For this review, take the finished solid that the model builds, in its own axes (mm). A direction names the side the tool comes from. Coordinates: 2 decimals unless noted, no trailing zeros. Loops run counter-clockwise (first coordinate to the right, second up) from the corner with the lowest first, then second, coordinate; pieces in that order, holes last. Notation, with made-up numbers: (26, 23.25) -> (74, 23.25) arc R23 ccw to (74, 59.25) -> close; hole circle Ø11 at (9.5, -30). An arc over 180 degrees is marked (long way). Answer in a Markdown table with one row per item.
from build123d import *
from build123d import SkipClean  # not in build123d's __all__

# Parameters (mm, degrees)
F1_DEPTH  = 10
F2_DEPTH  = 12.5
F3_DEPTH  = 10.3
F4_R      = 1.5
F5_DEPTH  = 2
F4_R_2    = 1.55
F6_DEPTH  = 5
F7_R      = 1.5
F8_DEPTH  = 2
F7_R_2    = 1.55
F9_DEPTH  = 5
F11_DEPTH = 12.5


with BuildPart() as f1:
    # F0 (on Front) → F1 (new body, symmetric)
    with BuildSketch(Plane.XZ):
        with BuildLine():
            ThreePointArc((0, -3.75), (2.6516504294, -2.6516504294), (3.75, 0))
            ThreePointArc((3.75, 0), (2.6516504294, 2.6516504294), (0, 3.75))
            ThreePointArc((0, 3.75), (-2.6516504294, 2.6516504294), (-3.75, 0))
            ThreePointArc((-3.75, 0), (-2.6516504294, -2.6516504294), (0, -3.75))
        make_face()
        with BuildLine():
            ThreePointArc((0, 3.75), (2.6516504294, 2.6516504294), (3.75, 0))
            ThreePointArc((3.75, 0), (4.8483495706, 2.6516504294), (7.5, 3.75))
            Line((7.5, 3.75), (0, 3.75))
        make_face()
        with BuildLine():
            ThreePointArc((7.5, 3.75), (4.8483495706, 2.6516504294), (3.75, 0))
            ThreePointArc((3.75, 0), (4.8483495706, -2.6516504294), (7.5, -3.75))
            ThreePointArc((7.5, -3.75), (10.1516504294, -2.6516504294), (11.25, 0))
            ThreePointArc((11.25, 0), (10.1516504294, 2.6516504294), (7.5, 3.75))
        make_face()
        with BuildLine():
            ThreePointArc((7.5, -3.75), (4.8483495706, -2.6516504294), (3.75, 0))
            ThreePointArc((3.75, 0), (2.6516504294, -2.6516504294), (0, -3.75))
            Line((0, -3.75), (7.5, -3.75))
        make_face()
    extrude(amount=F1_DEPTH, both=True)

    # F0 (on Front) → F2 (join, symmetric)
    with BuildSketch(Plane.XZ):
        with BuildLine():
            ThreePointArc((-7.5, -3.75), (-4.8483495706, -2.6516504294), (-3.75, 0))
            ThreePointArc((-3.75, 0), (-4.8483495706, 2.6516504294), (-7.5, 3.75))
            ThreePointArc((-7.5, 3.75), (-11.25, 0), (-7.5, -3.75))
        make_face()
        with BuildLine():
            ThreePointArc((-3.75, 0), (-2.6516504294, 2.6516504294), (0, 3.75))
            Line((0, 3.75), (-7.5, 3.75))
            ThreePointArc((-7.5, 3.75), (-4.8483495706, 2.6516504294), (-3.75, 0))
        make_face()
        with BuildLine():
            ThreePointArc((0, -3.75), (2.6516504294, -2.6516504294), (3.75, 0))
            ThreePointArc((3.75, 0), (2.6516504294, 2.6516504294), (0, 3.75))
            ThreePointArc((0, 3.75), (-2.6516504294, 2.6516504294), (-3.75, 0))
            ThreePointArc((-3.75, 0), (-2.6516504294, -2.6516504294), (0, -3.75))
        make_face()
        with BuildLine():
            Line((-7.5, -3.75), (0, -3.75))
            ThreePointArc((0, -3.75), (-2.6516504294, -2.6516504294), (-3.75, 0))
            ThreePointArc((-3.75, 0), (-4.8483495706, -2.6516504294), (-7.5, -3.75))
        make_face()
    extrude(amount=F2_DEPTH, both=True)

    # F0 (on Front) → F3 (cut, symmetric)
    with BuildSketch(Plane.XZ):
        with BuildLine():
            ThreePointArc((-7.5, -3.75), (-4.8483495706, -2.6516504294), (-3.75, 0))
            ThreePointArc((-3.75, 0), (-4.8483495706, 2.6516504294), (-7.5, 3.75))
            ThreePointArc((-7.5, 3.75), (-11.25, 0), (-7.5, -3.75))
        make_face()
        with BuildLine():
            Line((-7.5, -3.75), (0, -3.75))
            ThreePointArc((0, -3.75), (-2.6516504294, -2.6516504294), (-3.75, 0))
            ThreePointArc((-3.75, 0), (-4.8483495706, -2.6516504294), (-7.5, -3.75))
        make_face()
        with BuildLine():
            ThreePointArc((-3.75, 0), (-2.6516504294, 2.6516504294), (0, 3.75))
            Line((0, 3.75), (-7.5, 3.75))
            ThreePointArc((-7.5, 3.75), (-4.8483495706, 2.6516504294), (-3.75, 0))
        make_face()
    with SkipClean():  # cleaning this boolean's faces spoils the solid; the shape is the same uncleaned
        extrude(amount=F3_DEPTH, both=True, mode=Mode.SUBTRACT)

    # F4 (on face) → F5 (join)
    with BuildSketch(Plane.XZ.offset(10)):
        with Locations((7.5, 0)):
            Circle(F4_R)
    extrude(amount=F5_DEPTH)

    # F4 (on face) → F6 (cut)
    with BuildSketch(Plane.XZ.offset(10)):
        with Locations((-7.4913557619, 0)):
            Circle(F4_R_2)
    extrude(amount=F6_DEPTH, mode=Mode.SUBTRACT)

    # F7 (on face) → F8 (join)
    with BuildSketch(Plane(origin=(0, 10, 0), x_dir=(-1, 0, 0), z_dir=(0, 1, 0))):
        with Locations((-7.5, 0)):
            Circle(F7_R)
    extrude(amount=F8_DEPTH)

    # F7 (on face) → F9 (cut)
    with BuildSketch(Plane(origin=(0, 10, 0), x_dir=(-1, 0, 0), z_dir=(0, 1, 0))):
        with Locations((7.4891448021, 0)):
            Circle(F7_R_2)
    extrude(amount=F9_DEPTH, mode=Mode.SUBTRACT)

    # F10 (on Top) → F11 (cut, symmetric)
    with BuildSketch(Plane.XY):
        Polygon((-3.2, -10.3), (-3.2, 0), (-3.2, 10.3), (-14.7820527132, 10.3), (-14.7820527132, -10.3), align=None)
    extrude(amount=F11_DEPTH, both=True, mode=Mode.SUBTRACT)


solid = f1.part
Item 1: The part is to be moulded in two halves that separate along Y. For faces 5 (the flat face through (-3.2, 0, 0)), 6 (the flat face through (5.5, 10, 0.1)), 7 (the flat face through (-4, 11, -3.75)), say which applies: +Y half, -Y half, draft (parallel to the pull), parting line (faces both ways), or undercut.
Worked answers:
| item | result |
|---|---|
| face 5 | undercut |
| face 6 | +Y half |
| face 7 | draft |
Item 2: For faces 1 (the flat face through (-4, -11, -3.75)), 2 (the cylindrical face through (9, 11, 0)), 3 (the cylindrical face through (6, -11, 0)), 4 (the flat face through (7, -12, 0)), list the 3-axis set-ups (+Z, -Z, +X, -X, +Y, -Y) from which the entire face can be reached by the end or side of a thin tool; tool diameter is ignored.
Worked answers:
| item | result |
|---|---|
| face 1 | -Z, +X, -X, +Y, -Y |
| face 2 | +Y |
| face 3 | -Y |
| face 4 | +Z, -Z, +X, -Y |
Item 3: Take a section at A-A, the plane z = 0.75. State the section outline as (x, y) points.
Worked answers:
| item | result |
|---|---|
| outline | (-11.17, -12.5) -> (-8.85, -12.5) -> (-8.85, -10.3) -> (-11.17, -10.3) -> close; (-11.17, 10.3) -> (-8.85, 10.3) -> (-8.85, 12.5) -> (-11.17, 12.5) -> close; (-6.13, -12.5) -> (3.67, -12.5) -> (3.67, -10) -> (6.2, -10) -> (6.2, -12) -> (8.8, -12) -> (8.8, -10) -> (11.17, -10) -> (11.17, 10) -> (8.8, 10) -> (8.8, 12) -> (6.2, 12) -> (6.2, 10) -> (3.67, 10) -> (3.67, 12.5) -> (-6.13, 12.5) -> (-6.13, 10.3) -> (-3.2, 10.3) -> (-3.2, -10.3) -> (-6.13, -10.3) -> close |
Item 4: Take a section at C-C, the plane x = 1.75. State the section outline as (y, z) points, and give its area (3 significant figures).
Worked answers:
| item | result |
|---|---|
| outline | (-12.5, -3.32) -> (-10, -3.32) -> (-10, -3.75) -> (10, -3.75) -> (10, -3.32) -> (12.5, -3.32) -> (12.5, 3.32) -> (10, 3.32) -> (10, 3.75) -> (-10, 3.75) -> (-10, 3.32) -> (-12.5, 3.32) -> close |
| area | 183 mm² |
Item 5: Insertion check: pin 1 (3 mm diameter, centred on y = -3.5, z = 0, fed in from -X); pin 2 (4 mm diameter, centred on x = -7.49, z = 0, fed in from +Y); pin 3 (3.5 mm diameter, centred on x = 7.5, z = 0, fed in from -Y); pin 4 (3.5 mm diameter, centred on x = 7, z = 0.5, fed in from +Y). Each pin has a flat end and moves straight along its axis. Give the tip position at first contact, or say it passes through.
Worked answers:
| item | result |
|---|---|
| pin 1 | x = -3.2 |
| pin 2 | y = 12.5 |
| pin 3 | y = -12 |
| pin 4 | y = 12 |
Item 6: Take a section at B-B, the plane y = -1. State the section outline as (x, z) points.
Worked answers:
| item | result |
|---|---|
| outline | (-3.2, -1.96) arc R3.75 ccw to (0, -3.75) -> (7.5, -3.75) arc R3.75 ccw to (7.5, 3.75) -> (0, 3.75) arc R3.75 ccw to (-3.2, 1.96) -> close |
Item 7: Take a section at D-D, the plane z = -2.75. State the section outline as (x, y) points.
Worked answers:
| item | result |
|---|---|
| outline | (-10.05, -12.5) -> (2.55, -12.5) -> (2.55, -10) -> (10.05, -10) -> (10.05, 10) -> (2.55, 10) -> (2.55, 12.5) -> (-10.05, 12.5) -> (-10.05, 10.3) -> (-2.55, 10.3) -> (-2.55, -10.3) -> (-10.05, -10.3) -> close |
Item 8: For L1, parallel to Y at x = -3, z = 3.25; L2, parallel to Y at x = 6.5, z = -3.5; L3, parallel to X at y = 8, z = 3.25, list the stretches that pass through material, from the lowest coordinate up.
Worked answers:
| item | result |
|---|---|
| L1 | -12.5 to -10.3, 10.3 to 12.5 |
| L2 | -10 to 10 |
| L3 | -1.87 to 9.37 |
